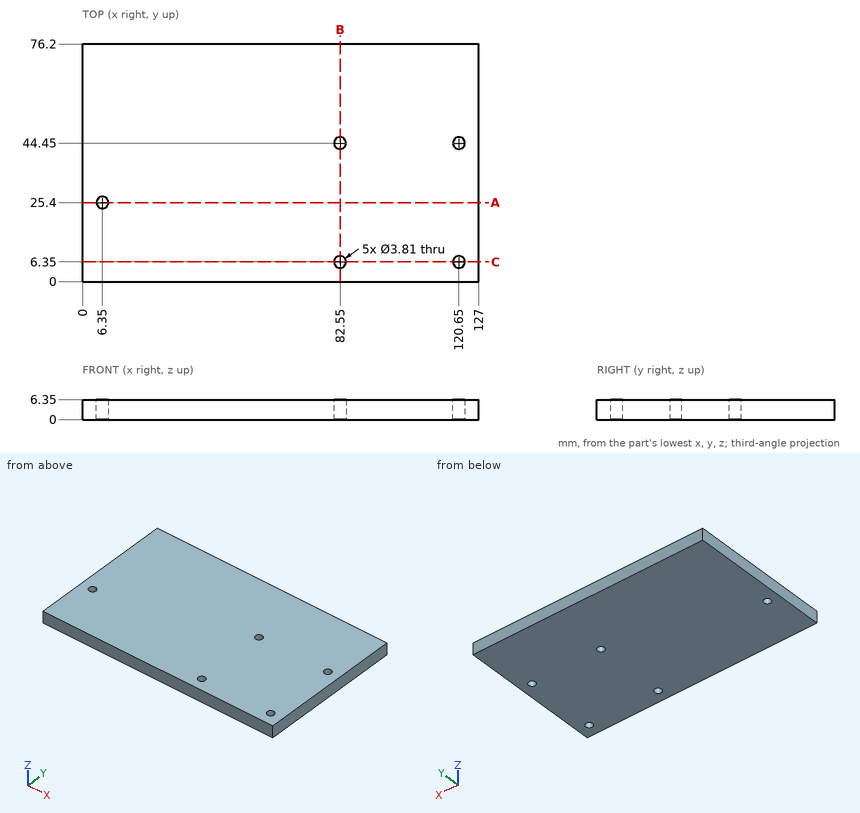
Study the drawing (mm; zero at the part's minimum x, y, z) and answer. Give positions to 0.01 mm unless a question says otherwise; leave off trailing zeros. Write each loop counter-clockwise with the first axis right and the second up, starting at its lowest first coordinate (ties: lowest second). Pieces come first, ordered by that corner, then holes. Notation, with made-up numbers: (-20.5, -38.75) -> (34.5, -38.75) arc R23 cw to (34.5, -13.75) -> close; hole circle Ø6 at (87, -3). An arc over 180 degrees is marked (long way). Answer as a JSON object with one key per item and string values. Group by question number.
1) Find section C-C (y = 6.35). Write down the section's boundary in (x, z) (3 decimals).
2) Find section A-A (y = 25.4). Write down the section's boundary in (x, z) (3 decimals), and give its area (3 significant figures).
3) Find section B-B (x = 82.55). Write down the section's boundary in (y, z) (3 decimals).
4) Consider L1, parallel to X at y = 44.45, z = 5.25 (3 decimals); L2, parallel to Y at x = 120.65, z = 3 (3 decimals); L3, parallel to Y at x = 6.35, z = 3 (3 decimals). Determine where each line is inside the solid, lowest interval first. Write a range as from..to.
Values follow:
{
 "1": {"outline": "(0, 0) -> (80.645, 0) -> (80.645, 6.35) -> (0, 6.35) -> close; (84.455, 0) -> (118.745, 0) -> (118.745, 6.35) -> (84.455, 6.35) -> close; (122.555, 0) -> (127, 0) -> (127, 6.35) -> (122.555, 6.35) -> close"},
 "2": {"outline": "(0, 0) -> (4.445, 0) -> (4.445, 6.35) -> (0, 6.35) -> close; (8.255, 0) -> (127, 0) -> (127, 6.35) -> (8.255, 6.35) -> close", "area": "782 mm2"},
 "3": {"outline": "(0, 0) -> (4.445, 0) -> (4.445, 6.35) -> (0, 6.35) -> close; (8.255, 0) -> (42.545, 0) -> (42.545, 6.35) -> (8.255, 6.35) -> close; (46.355, 0) -> (76.2, 0) -> (76.2, 6.35) -> (46.355, 6.35) -> close"},
 "4": {"L1": "x = 0..80.645, 84.455..118.745, 122.555..127", "L2": "y = 0..4.445, 8.255..42.545, 46.355..76.2", "L3": "y = 0..23.495, 27.305..76.2"}
}
